```python
from build123d import *

# Parameters (mm, degrees)
BOSS_EXTRUDE1_DEPTH = 18.25625
SKETCH4_W           = 88.9
SKETCH4_H           = 88.9
BOSS_EXTRUDE2_DEPTH = 18.25625
FILLET1_R           = 3.3782


with BuildPart() as part:
    # Sketch3 → Boss-Extrude1 (new body)
    with BuildSketch(Plane(origin=(0, 0, 0), x_dir=(1, 0, 0), z_dir=(0, 1, 0))):
        with BuildLine():
            Line((-501.65, -501.65), (-590.55, -590.55))
            Line((-590.55, -590.55), (-553.84414606, -590.55))
            ThreePointArc((-553.84414606, -590.55), (0, -809.625), (553.84414606, -590.55))
            Line((553.84414606, -590.55), (590.55, -590.55))
            Line((590.55, -590.55), (501.65, -501.65))
            Line((501.65, -501.65), (501.65, -569.352841501))
            ThreePointArc((501.65, -569.352841501), (0, -758.825), (-501.65, -569.352841501))
            Line((-501.65, -569.352841501), (-501.65, -501.65))
        make_face()
    extrude(amount=BOSS_EXTRUDE1_DEPTH)

    # Sketch4 → Boss-Extrude2 (add)
    with BuildSketch(Plane(origin=(0, 18.25625, 0), x_dir=(1, 0, 0), z_dir=(0, 1, 0))):
        with Locations((-546.1, -546.1)):
            Rectangle(SKETCH4_W, SKETCH4_H)
        with Locations((546.1, -546.1)):
            Rectangle(SKETCH4_W, SKETCH4_H)
    extrude(amount=-BOSS_EXTRUDE2_DEPTH)

    # Fillet1
    fillet1_edges = [part.edges().sort_by_distance(p)[0] for p in [
        (-501.65, 9.128125, 569.352841501),
        (501.65, 9.128125, 569.352841501),
        (553.84414606, 9.128125, 590.55),
        (-553.84414606, 9.128125, 590.55),
    ]]
    fillet(fillet1_edges, radius=FILLET1_R)


solid = part.part
```
Geometry check sheet. Reference: the model listing, model coordinates, mm. Coordinates: 2 decimals unless noted, no trailing zeros. Order: outer loops, then holes, each group sorted by start corner. A loop starts at its lowest first (then second) coordinate and runs counter-clockwise, first axis right, second up.
Q1. Draft check along X on faces 1 (the face through (-3, 0, 769)), 2 (the face through (-8.52, 9, 809.58)), 3 (the face through (7.651, 9, 758.786)). Enter one of: released by +X, released by -X, zero draft, split by the parting line, or undercut.
Reply:
face 1: zero draft
face 2: split by the parting line
face 3: undercut
Q2. Depth check by flat-ended pin: pin 1 Ø3 at (x, y) = (-269.5, 14) entering from -Z; pin 2 Ø5 at (x, y) = (193, 6) entering from +Z; pin 3 Ø1 at (x, y) = (-387.5, 7) entering from +Z. Enter the tip coordinate at first touch or a pass-through.
Reply:
pin 1: stops at z = 708.78
pin 2: stops at z = 786.89
pin 3: stops at z = 711.14
Q3. Sectioned sample at C-C on z = 608. Record the cut outline in (x, y), and give its area (3 significant figures).
Reply:
outline: (-534.63, 0) - (-454.04, 0) - (-454.04, 18.26) - (-534.63, 18.26) - close; (454.04, 0) - (534.63, 0) - (534.63, 18.26) - (454.04, 18.26) - close
area: 2,940 mm2
Q4. Sectioned sample at B-B on y = 3. Record the cut outline in (x, z) (3 decimals), and give its area (3 significant figures).
Reply:
outline: (-590.55, 501.65) - (-501.65, 501.65) - (-501.65, 567.825) arc R3.378 cw to (-500.5, 570.364) arc R758.825 cw to (500.5, 570.364) arc R3.378 cw to (501.65, 567.825) - (501.65, 501.65) - (590.55, 501.65) - (590.55, 590.55) - (555.179, 590.55) arc R3.378 cw to (552.872, 591.46) arc R809.625 ccw to (-552.872, 591.46) arc R3.378 cw to (-555.179, 590.55) - (-590.55, 590.55) - close
area: 73,500 mm2
Q5. Sectioned sample at D-D on x = 136.5. Record the cut outline in (y, z), and give its area (3 significant figures).
Reply:
outline: (0, 746.45) - (18.26, 746.45) - (18.26, 798.04) - (0, 798.04) - close
area: 942 mm2
Q6. Thickness scan on probe 1 along X at (y, z) = (9.5, 547.5); probe 2 along X at (y, z) = (7.75, 664); probe 3 along Z at (x, y) = (4.5, 15). Record the ranges inside material, lowest first.
Reply:
probe 1: x = -590.55 to -501.65, 501.65 to 590.55
probe 2: x = -463.25 to -367.31, 367.31 to 463.25
probe 3: z = 758.81 to 809.61
Q7. Sectioned sample at A-A on z = 533. Record the cut outline in (x, y).
Reply:
outline: (-590.55, 0) - (-501.65, 0) - (-501.65, 18.26) - (-590.55, 18.26) - close; (501.65, 0) - (590.55, 0) - (590.55, 18.26) - (501.65, 18.26) - close
